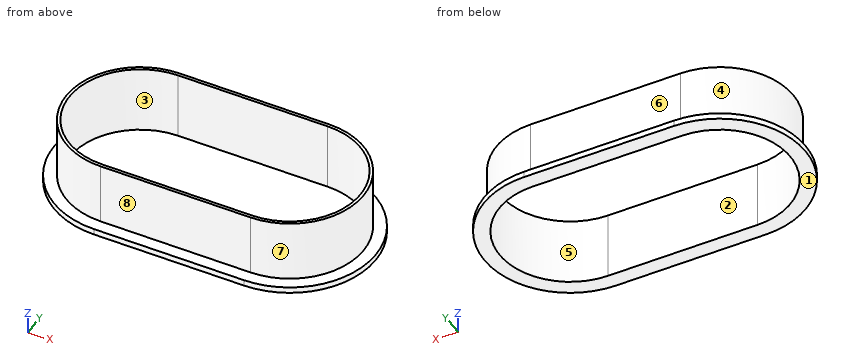
from build123d import *

# Parameters (mm, degrees)
F1_DEPTH = 2
F2_DEPTH = 20.5


with BuildPart() as f1:
    # F0 (on Top) → F1 (new body)
    with BuildSketch(Plane.XY):
        with BuildLine():
            Line((49, 28), (0, 28))
            ThreePointArc((0, 28), (-28, 0), (0, -28))
            Line((0, -28), (49, -28))
            ThreePointArc((49, -28), (77, 0), (49, 28))
        make_face()
        with BuildLine():
            ThreePointArc((0, -24), (-24, 0), (0, 24))
            Line((0, 24), (49, 24))
            ThreePointArc((49, 24), (73, 0), (49, -24))
            Line((49, -24), (0, -24))
        make_face(mode=Mode.SUBTRACT)
        with BuildLine():
            Line((49, 24), (0, 24))
            ThreePointArc((0, 24), (-24, 0), (0, -24))
            Line((0, -24), (49, -24))
            ThreePointArc((49, -24), (73, 0), (49, 24))
        make_face()
        with BuildLine():
            ThreePointArc((0, -23), (-23, 0), (0, 23))
            Line((0, 23), (49, 23))
            ThreePointArc((49, 23), (72, 0), (49, -23))
            Line((49, -23), (0, -23))
        make_face(mode=Mode.SUBTRACT)
    extrude(amount=-F1_DEPTH)

    # F0 (on Top) → F2 (join)
    with BuildSketch(Plane.XY):
        with BuildLine():
            Line((49, 24), (0, 24))
            ThreePointArc((0, 24), (-24, 0), (0, -24))
            Line((0, -24), (49, -24))
            ThreePointArc((49, -24), (73, 0), (49, 24))
        make_face()
        with BuildLine():
            ThreePointArc((0, -23), (-23, 0), (0, 23))
            Line((0, 23), (49, 23))
            ThreePointArc((49, 23), (72, 0), (49, -23))
            Line((49, -23), (0, -23))
        make_face(mode=Mode.SUBTRACT)
    extrude(amount=F2_DEPTH)


solid = f1.part
Can you work these out from the model? Positions are in its coordinate system, mm. Face numbers are marked on the shaded views. A direction names the side the tool comes from. Coordinates: 2 decimals unless noted, no trailing zeros. Write each loop counter-clockwise with the first axis right and the second up, starting at its lowest first coordinate (ties: lowest second). Pieces come first, ordered by that corner, then holes. Notation, with made-up numbers: (61, -27.5) - (84, -27.5) arc R25 cw to (84, -12.5) - close; hole circle Ø10 at (-31, 3.25). An arc over 180 degrees is marked (long way). Return JSON: item names as keys, results as strings. Group by question number.
Item 1: If we section it at B-B (x = 45.5): Write out the boundary of the cut face in (y, z), then the cut area to 3 significant figures.
Item 2: If we section it at C-C (z = 6.75): Write out the boundary of the cut face in (x, y), then the cut area to 3 significant figures.
Item 3: I'm going to push flat-ended pins straight in: pin 1 Ø4 at (x, z) = (26.5, 8) entering from -Y; pin 2 Ø3 at (y, z) = (17, 6) entering from +X; pin 3 Ø8 at (y, z) = (-11.5, 0.5) entering from +X. Where does each tip first touch, or does it pass through?
Item 4: We'd pull the mould along X, two halves only. Please class the marked faces 1, 2, 3 and 4: pulls with the +X half, pulls with the -X half, needs draft (parallel to the pull), parting line crosses it, or undercut.
Item 5: Please list where these lines run through material, in increasing order: probe 1 along Y at (x, z) = (37.5, 19.5); probe 2 along Y at (x, z) = (-2, 12); probe 3 along X at (y, z) = (-18, 5.25).
Item 6: Which directions (+Z, -Z, +X, -X, +Y, -Y) give clear straight access to the entire face, cutting with the end or side of a thin tool? Please do the marked faces 5, 6, 7 and 8.
Item 7: If we section it at A-A (y = 0): Write out the boundary of the cut face in (x, z), then the cut area to 3 significant figures.
Return value:
{
 "1": {"outline": "(-28, -2) - (-23, -2) - (-23, 20.5) - (-24, 20.5) - (-24, 0) - (-28, 0) - close; (23, -2) - (28, -2) - (28, 0) - (24, 0) - (24, 20.5) - (23, 20.5) - close", "area": "61.0 mm^2"},
 "2": {"outline": "(0, -24) - (49, -24) arc R24 ccw to (49, 24) - (0, 24) arc R24 ccw to start; hole (0, -23) - (49, -23) arc R23 ccw to (49, 23) - (0, 23) arc R23 ccw to start", "area": "246 mm^2"},
 "3": {"pin 1": "stops at y = -24", "pin 2": "stops at x = 67.32", "pin 3": "stops at x = 75.97"},
 "4": {"face 1": "needs draft", "face 2": "undercut", "face 3": "undercut", "face 4": "pulls with the -X half"},
 "5": {"probe 1": "y = -24 to -23, 23 to 24", "probe 2": "y = -23.92 to -22.91, 22.91 to 23.92", "probe 3": "x = -15.87 to -14.32, 63.32 to 64.87"},
 "6": {"face 5": "+Z, -Z", "face 6": "+Z, +X, -X, +Y", "face 7": "+Z, +X", "face 8": "+Z, +X, -X, -Y"},
 "7": {"outline": "(-28, -2) - (-23, -2) - (-23, 20.5) - (-24, 20.5) - (-24, 0) - (-28, 0) - close; (72, -2) - (77, -2) - (77, 0) - (73, 0) - (73, 20.5) - (72, 20.5) - close", "area": "61.0 mm^2"}
}
